from build123d import *

# Parameters (mm, degrees)
F0_W     = 125
F0_H     = 25
F1_DEPTH = 100
F3_DEPTH = 50


with BuildPart() as f1:
    # F0 (on Top) → F1 (new body)
    with BuildSketch(Plane.XY):
        Rectangle(F0_W, F0_H)
    extrude(amount=F1_DEPTH)

    # F2 (on face) → F3 (join)
    with BuildSketch(Plane.XY.offset(100)):
        with BuildLine():
            Line((-3.9200801402, 9), (-3.9200801402, 11))
            ThreePointArc((-3.9200801402, 11), (-14.9200801402, 0), (-3.9200801402, -11))
            Line((-3.9200801402, -11), (-3.9200801402, -9))
            ThreePointArc((-3.9200801402, -9), (-12.9200801402, 0), (-3.9200801402, 9))
        make_face()
        with BuildLine():
            ThreePointArc((7.0799198598, 0), (3.8580944528, 7.7781745931), (-3.9200801402, 11))
            Line((-3.9200801402, 11), (-3.9200801402, 9))
            ThreePointArc((-3.9200801402, 9), (2.4438808904, 6.3639610307), (5.0799198598, 0))
            ThreePointArc((5.0799198598, 0), (2.4438808904, -6.3639610307), (-3.9200801402, -9))
            Line((-3.9200801402, -9), (-3.9200801402, -11))
            ThreePointArc((-3.9200801402, -11), (3.8580944528, -7.7781745931), (7.0799198598, 0))
        make_face()
    extrude(amount=F3_DEPTH)


solid = f1.part
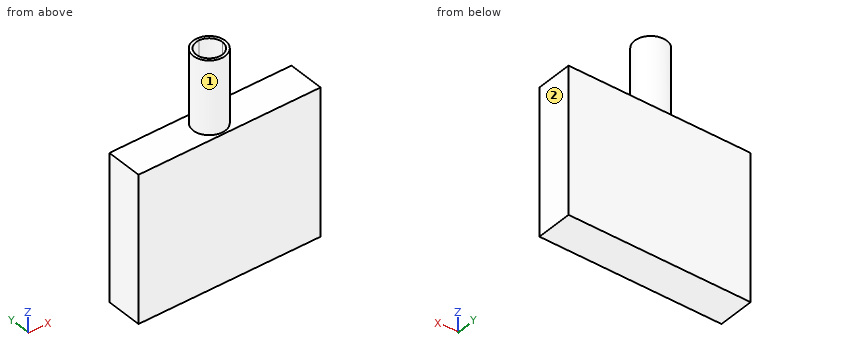
Input: part model. Units: mm. Frame: model coordinates. Face numbers are marked on the shaded views. A direction names the side the tool comes from. Round coordinates to 2 decimals unless told otherwise and drop trailing zeros. Order: outer loops, then holes, each group sorted by start corner. A loop starts at its lowest first (then second) coordinate and runs counter-clockwise, first axis right, second up. Notation, with made-up numbers: (11.25, 16) - (51.25, 16) arc R33 cw to (51.25, 50) - close; hole circle Ø5 at (67, -7). An arc over 180 degrees is marked (long way). Answer as a JSON object with one key per item and string values. Group by question number.
(1) Reachability of the marked faces 1 and 2 from +Z, -Z, +X, -X, +Y, -Y: full face, straight path, thin tool, end or side. Return the list, or none.
(2) Cut plane C-C (x = 23.5). Return loops of the section in (y, z), then the cut area to 3 significant figures.
(3) Cut plane A-A (x = 1). Return loops of the section in (y, z), then the cut area to 3 significant figures.
(4) Material intervals for probe 1 along Z at (x, y) = (-11, 4.75); probe 2 along Y at (x, z) = (3.5, 128); probe 3 along X at (y, z) = (-3.5, 102.5), sorted ascending. Write a range as from..to.
(5) Cut plane B-B (y = -2). Return loops of the section in (x, z).
(6) Pin query (flat end, axial travel): P1, Ø5.5, axis at x = -8, y = 3, coming from the +Z side. Return the tip coordinate at first contact, or that it passes through.
Here are the results:
{
 "1": {"face 1": "+Z", "face 2": "+Z, -Z, +X, +Y, -Y"},
 "2": {"outline": "(-12.5, 0) - (12.5, 0) - (12.5, 100) - (-12.5, 100) - close", "area": "2,500 mm^2"},
 "3": {"outline": "(-12.5, 0) - (12.5, 0) - (12.5, 100) - (9.84, 100) - (9.84, 150) - (7.54, 150) - (7.54, 100) - (-7.54, 100) - (-7.54, 150) - (-9.84, 150) - (-9.84, 100) - (-12.5, 100) - close", "area": "2,730 mm^2"},
 "4": {"probe 1": "z = 0..100", "probe 2": "y = -8.12..-5.09, 5.09..8.12", "probe 3": "x = -14.35..-12.21, 4.37..6.51"},
 "5": {"outline": "(-62.5, 0) - (62.5, 0) - (62.5, 100) - (6.9, 100) - (6.9, 150) - (4.85, 150) - (4.85, 100) - (-12.7, 100) - (-12.7, 150) - (-14.74, 150) - (-14.74, 100) - (-62.5, 100) - close"},
 "6": {"P1": "stops at z = 100"}
}
